Can you work these out from the model? Positions are in its coordinate system, mm. A direction names the side the tool comes from. Give positions to 0.01 mm unless a question says otherwise; leave off trailing zeros. Loops run counter-clockwise (first coordinate to the right, second up) from the corner with the lowest first, then second, coordinate; pieces in that order, holes last. Notation, with made-up numbers: (-4, -10.75) - (38, -10.75) arc R20 ccw to (38, 21.25) - close; hole circle Ø9 at (24.5, -23.5). An arc over 180 degrees is marked (long way). Answer in a Markdown table with one row per item.
from build123d import *

# Parameters (mm, degrees)
F0_R     = 70.804177
F0_R_2   = 60.644177
F1_DEPTH = 9.906
F2_DEPTH = 12.7
F3_DEPTH = 15.24


with BuildPart() as f1:
    # F0 (on Front) → F1 (new body, symmetric)
    with BuildSketch(Plane.XZ):
        Circle(F0_R)
        Circle(F0_R_2, mode=Mode.SUBTRACT)
    extrude(amount=F1_DEPTH, both=True)

    # F0 (on Front) → F2 (join, symmetric)
    with BuildSketch(Plane.XZ):
        Circle(F0_R_2)
        Polygon((-6.35, 0), (-26.848431, 41.6581), (26.848444, 41.6581), (6.35, 0), (26.84843, -41.658109), (-26.84843, -41.658109), align=None, mode=Mode.SUBTRACT)
    extrude(amount=F2_DEPTH, both=True)

    # F0 (on Front) → F3 (join)
    with BuildSketch(Plane.XZ):
        Polygon((26.848444, 41.6581), (-26.848431, 41.6581), (-6.35, 0), (-26.84843, -41.658109), (26.84843, -41.658109), (6.35, 0), align=None)
    extrude(amount=F3_DEPTH)


solid = f1.part
Q1. Imagine slicing it at B-B, the plane z = 44. Write out the boundary of the cut face in (x, y), and give its area (3 significant figures).
Checked values:
| item | result |
|---|---|
| outline | (-55.47, -9.91) - (-41.73, -9.91) - (-41.73, -12.7) - (41.73, -12.7) - (41.73, -9.91) - (55.47, -9.91) - (55.47, 9.91) - (41.73, 9.91) - (41.73, 12.7) - (-41.73, 12.7) - (-41.73, 9.91) - (-55.47, 9.91) - close |
| area | 2,660 mm² |
Q2. If I drill on line 1 (Z direction, x = -14, y = 8.5); line 2 (Z direction, x = -0.5, y = 0.75); line 3 (Y direction, x = -21, z = 49), over which ranges is the centre line in solid material (lowest first)? Write a range as [from, to].
Checked values:
| item | result |
|---|---|
| line 1 | z = [-69.41, -41.66], [-15.55, 15.55], [41.66, 69.41] |
| line 2 | z = [-70.8, -41.66], [41.66, 70.8] |
| line 3 | y = [-12.7, 12.7] |
Q3. Imagine slicing it at D-D, the plane x = -45. Write out the boundary of the cut face in (y, z).
Checked values:
| item | result |
|---|---|
| outline | (-12.7, -40.65) - (-9.91, -40.65) - (-9.91, -54.66) - (9.91, -54.66) - (9.91, -40.65) - (12.7, -40.65) - (12.7, 40.65) - (9.91, 40.65) - (9.91, 54.66) - (-9.91, 54.66) - (-9.91, 40.65) - (-12.7, 40.65) - close |
Q4. If we mould it in two halves opening along X, with no side actions, what happens to faces 6 (the face through (-16.456, 6.261, 20.537)), 7 (the face through (16.743, -13.952, -21.121)), 8 (the face through (13, -12.7, 1))? For each: released by +X, released by -X, zero draft, split by the parting line, or undercut.
Checked values:
| item | result |
|---|---|
| face 6 | undercut |
| face 7 | released by +X |
| face 8 | zero draft |
Q5. Imagine slicing it at C-C, the plane x = 0. Write out the boundary of the cut face in (y, z).
Checked values:
| item | result |
|---|---|
| outline | (-15.24, -41.66) - (-12.7, -41.66) - (-12.7, -60.64) - (-9.91, -60.64) - (-9.91, -70.8) - (9.91, -70.8) - (9.91, -60.64) - (12.7, -60.64) - (12.7, -41.66) - (0, -41.66) - (0, 41.66) - (12.7, 41.66) - (12.7, 60.64) - (9.91, 60.64) - (9.91, 70.8) - (-9.91, 70.8) - (-9.91, 60.64) - (-12.7, 60.64) - (-12.7, 41.66) - (-15.24, 41.66) - close |
Q6. Imagine slicing it at A-A, the plane y = 2. Write out the boundary of the cut face in (x, z).
Checked values:
| item | result |
|---|---|
| outline | circle Ø141.61 at (0, 0); hole (-26.85, -41.66) - (26.85, -41.66) - (6.35, 0) - (26.85, 41.66) - (-26.85, 41.66) - (-6.35, 0) - close |
Q7. For pin 1 (4 mm diameter, centred on y = -3, z = -35, fed in from -X); pin 2 (6.5 mm diameter, centred on x = -6.5, y = 5.5, fed in from -Z); pin 3 (1 mm diameter, centred on x = -27, z = -4, fed in from -Y), each with a flat end and sliding along its axis, tell me the tip position at first contact or that it passes through.
Checked values:
| item | result |
|---|---|
| pin 1 | stops at x = -62.64 |
| pin 2 | stops at z = -70.73 |
| pin 3 | stops at y = -12.7 |
Q8. On a 3-axis mill with a long thin cutter (end or side, diameter ignored), from which of +Z, -Z, +X, -X, +Y, -Y can I reach the whole of each face in a straight line? I mean faces 1 (the face through (16.456, -13.952, 20.537)), 2 (the face through (0, 0, 1)), 3 (the face through (-9.22, -0.14, 70.2)), 4 (the face through (-16.743, -13.952, 21.121)), 5 (the face through (52, -9.906, 32)). Say none if no direction works.
Checked values:
| item | result |
|---|---|
| face 1 | +X, -Y |
| face 2 | +Y |
| face 3 | +Y, -Y |
| face 4 | -X, -Y |
| face 5 | -Y |
